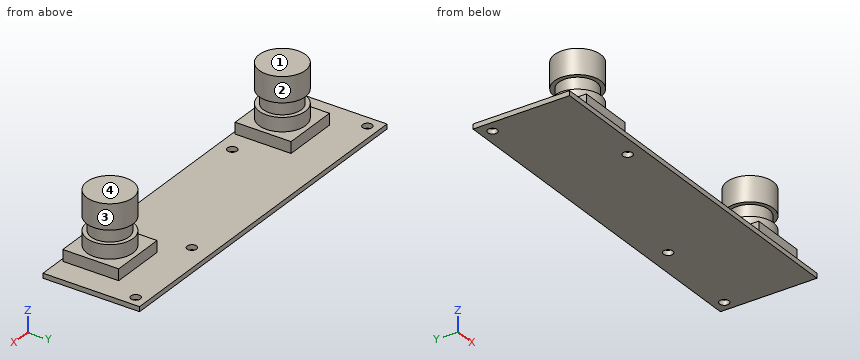
from build123d import *

# Parameters (mm, degrees)
SKETCH1_W           = 86
SKETCH1_H           = 23
BOSS_EXTRUDE1_DEPTH = 1.15
SKETCH2_W           = 13.35
SKETCH2_H           = 13.31
BOSS_EXTRUDE2_DEPTH = 2.7
SKETCH3_R           = 5.5
BOSS_EXTRUDE3_DEPTH = 3.3
SKETCH5_R           = 4.5
BOSS_EXTRUDE4_DEPTH = 3.3
SKETCH6_R           = 5.5
BOSS_EXTRUDE5_DEPTH = 6
SKETCH7_R           = 1.125
CUT_EXTRUDE1_DEPTH  = 3


with BuildPart() as part:
    # Sketch1 → Boss-Extrude1 (new body)
    with BuildSketch(Plane.XY):
        Rectangle(SKETCH1_W, SKETCH1_H)
    extrude(amount=-BOSS_EXTRUDE1_DEPTH)

    # Sketch2 → Boss-Extrude2 (add)
    with BuildSketch(Plane.XY):
        with Locations((-29.585, -4.237161914)):
            Rectangle(SKETCH2_W, SKETCH2_H)
        with Locations((30.325, -4.237161914)):
            Rectangle(SKETCH2_W, SKETCH2_H)
    extrude(amount=BOSS_EXTRUDE2_DEPTH)

    # Sketch3 → Boss-Extrude3 (add)
    with BuildSketch(Plane.XY.offset(2.7)):
        with Locations((-29.585, -4.237161914)):
            Circle(SKETCH3_R)
    boss_extrude3 = extrude(amount=BOSS_EXTRUDE3_DEPTH)

    # Sketch5 → Boss-Extrude4 (add)
    with BuildSketch(Plane.XY.offset(6)):
        with Locations((-29.585, -4.237161914)):
            Circle(SKETCH5_R)
    boss_extrude4 = extrude(amount=BOSS_EXTRUDE4_DEPTH)

    # Sketch6 → Boss-Extrude5 (add)
    with BuildSketch(Plane.XY.offset(9.3)):
        with Locations((-29.585, -4.237161914)):
            Circle(SKETCH6_R)
    boss_extrude5 = extrude(amount=BOSS_EXTRUDE5_DEPTH)

    # Mirror1: Boss-Extrude3, Boss-Extrude4, Boss-Extrude5 across plane
    add(boss_extrude3.mirror(Plane(origin=(0.37, 0, 0), x_dir=(0, 0, 1), z_dir=(1, 0, 0))))
    add(boss_extrude4.mirror(Plane(origin=(0.37, 0, 0), x_dir=(0, 0, 1), z_dir=(1, 0, 0))))
    add(boss_extrude5.mirror(Plane(origin=(0.37, 0, 0), x_dir=(0, 0, 1), z_dir=(1, 0, 0))))

    # Sketch7 → Cut-Extrude1 (cut)
    with BuildSketch(Plane(origin=(0, 0, -1.15), x_dir=(-1, 0, 0), z_dir=(0, 0, -1))):
        with Locations((40.175, 8.775)):
            Circle(SKETCH7_R)
        with Locations((17.685, -7.995)):
            Circle(SKETCH7_R)
        with Locations((-18.245, 6.995)):
            Circle(SKETCH7_R)
        with Locations((-40.445, 8.835764466)):
            Circle(SKETCH7_R)
    extrude(amount=-CUT_EXTRUDE1_DEPTH, mode=Mode.SUBTRACT)


solid = part.part
Model file for the job. Use its own axes, mm. Face numbers are marked on the shaded views. A direction names the side the tool comes from. Coordinates: 2 decimals unless noted, no trailing zeros. Loops run counter-clockwise (first coordinate to the right, second up) from the corner with the lowest first, then second, coordinate; pieces in that order, holes last. Notation, with made-up numbers: (-3.5, 3.5) -> (34.5, 3.5) arc R36 ccw to (34.5, 41.5) -> close; hole circle Ø5 at (30, 72.5). An arc over 180 degrees is marked (long way). Use one line per item in the form item = value. Start each with the question number.
(1) Probe probe 1 along Z at (x, y) = (7, 0); probe 2 along X at (y, z) = (-4.5, 3.5); probe 3 along X at (y, z) = (-3.25, 9.5). List the from-to ranges inside material, lowest first. Write a range as from..to.
(2) Cut at A-A on z = 0.75. Give the cut face in (x, y).
(3) Cut at B-B on x = -13.5. Give the cut face in (y, z), and give its area (4 significant figures).
(4) Flat gauge pins, fed straight in: pin 1 (2.5 mm diameter, centred on x = 18.245, y = 6.995, fed in from +Z); pin 2 (1.4 mm diameter, centred on y = -3, z = 1, fed in from +X); pin 3 (1.4 mm diameter, centred on x = 31, z = 1, fed in from +Y). Where does each tip first touch, or does it go through?
(5) Tool access for the marked faces 3 and 4: list every direction of +Z, -Z, +X, -X, +Y, -Y with a clear straight run to the whole face (end or side of a thin tool).
(6) Pull direction X, two halves, no side cores. Call the marked faces 1 and 2: pulls with the +X half, pulls with the -X half, needs draft (parallel to the pull), parting line crosses it, or undercut.
(7) Cut at D-D on x = -32.5. Give the cut face in (y, z).
(8) Cut at C-C on y = 5. Give the cut face in (x, z), and give its area (3 significant figures).
Values:
q1.probe_1 = -1.15..0
q1.probe_2 = -35.08..-24.09, 24.83..35.82
q1.probe_3 = -35..-24.17, 24.91..35.74
q2.outline = (-36.26, -10.89) -> (-22.91, -10.89) -> (-22.91, 2.42) -> (-36.26, 2.42) -> close; (23.65, -10.89) -> (37, -10.89) -> (37, 2.42) -> (23.65, 2.42) -> close
q3.outline = (-11.5, -1.15) -> (11.5, -1.15) -> (11.5, 0) -> (-11.5, 0) -> close
q3.area = 26.45 mm2
q4.pin_1 = 0
q4.pin_2 = 37
q4.pin_3 = 2.42
q5.face_3 = +Z
q5.face_4 = +Z, +X, -X, +Y, -Y
q6.face_1 = needs draft
q6.face_2 = undercut
q7.outline = (-11.5, -1.15) -> (11.5, -1.15) -> (11.5, 0) -> (2.42, 0) -> (2.42, 2.7) -> (0.43, 2.7) -> (0.43, 6) -> (-0.81, 6) -> (-0.81, 9.3) -> (0.43, 9.3) -> (0.43, 15.3) -> (-8.9, 15.3) -> (-8.9, 9.3) -> (-7.67, 9.3) -> (-7.67, 6) -> (-8.9, 6) -> (-8.9, 2.7) -> (-10.89, 2.7) -> (-10.89, 0) -> (-11.5, 0) -> close
q8.outline = (-43, -1.15) -> (43, -1.15) -> (43, 0) -> (-43, 0) -> close
q8.area = 98.9 mm2
